Could you check a few things on this model? Use its own coordinates, in mm. Face numbers are marked on the shaded views. A direction names the side the tool comes from. Round coordinates to 2 decimals unless told otherwise and drop trailing zeros. Write each loop counter-clockwise with the first axis right and the second up, starting at its lowest first coordinate (ties: lowest second). Pieces come first, ordered by that corner, then holes. Notation, with made-up numbers: (-24.5, 17.5) -> (20.5, 17.5) arc R12 cw to (20.5, 31.5) -> close; hole circle Ø4 at (75, 78). An arc over 180 degrees is marked (long way). Answer in a Markdown table with one row per item.
from build123d import *

# Parameters (mm, degrees)
SKETCH2_R           = 25
BOSS_EXTRUDE1_DEPTH = 10
SKETCH3_R           = 17.5
BOSS_EXTRUDE3_DEPTH = 20
SKETCH4_R           = 13.5
CUT_EXTRUDE1_DEPTH  = 25
SKETCH5_W           = 13.75
SKETCH5_H           = 13.75
BOSS_EXTRUDE4_DEPTH = 100
FILLET2_R           = 2.5
FILLET3_R           = 2.5
WRAP1_START         = 12.5
WRAP1_OUTLINE_R     = 18
WRAP1_OUTLINE_R_2   = 17.5
WRAP1_DEPTH         = 6.23469337
SKETCH8_W           = 13.75
SKETCH8_H           = 13.75
CUT_EXTRUDE2_DEPTH  = 5
SKETCH8_2_W         = 13.75
SKETCH8_2_H         = 13.75
CUT_EXTRUDE3_DEPTH  = 10
SCALE1_SCALE        = 0.8


# Read off the part's stored shape, not the designer's step: Wrap1
with BuildPart() as part:
    # Sketch2 → Boss-Extrude1 (new body)
    with BuildSketch(Plane(origin=(0, 0, 0), x_dir=(1, 0, 0), z_dir=(0, 1, 0))):
        with Locations(Location((0, 0, 0), (0, 0, 270))):
            Circle(SKETCH2_R)
    extrude(amount=BOSS_EXTRUDE1_DEPTH)

    # Sketch3 → Boss-Extrude3 (add)
    with BuildSketch(Plane(origin=(0, 10, 0), x_dir=(1, 0, 0), z_dir=(0, 1, 0))):
        with Locations(Location((0, 0, 0), (0, 0, 270))):
            Circle(SKETCH3_R)
    extrude(amount=BOSS_EXTRUDE3_DEPTH)

    # Sketch4 → Cut-Extrude1 (cut)
    with BuildSketch(Plane(origin=(0, 30, 0), x_dir=(1, 0, 0), z_dir=(0, 1, 0))):
        with Locations(Location((0, 0, 0), (0, 0, 270))):
            Circle(SKETCH4_R)
    extrude(amount=-CUT_EXTRUDE1_DEPTH, mode=Mode.SUBTRACT)

    # Sketch5 → Boss-Extrude4 (add)
    with BuildSketch(Plane.XZ):
        Rectangle(SKETCH5_W, SKETCH5_H)
    extrude(amount=BOSS_EXTRUDE4_DEPTH)

    # Fillet2
    fillet2_edges = [part.edges().sort_by_distance(p)[0] for p in [
        (0, 0, -25),
        (0, 10, -25),
        (0, 10, -17.5),
    ]]
    fillet(fillet2_edges, radius=FILLET2_R)

    # Fillet3
    fillet3_edges = [part.edges().sort_by_distance(p)[0] for p in [
        (0, 30, -17.5),
    ]]
    fillet(fillet3_edges, radius=FILLET3_R)

    # Wrap1 outline → Wrap1 (add)
    with BuildSketch(Plane(origin=(0, 0, 0), x_dir=(1, 0, 0), z_dir=(0, 1, 0)).offset(WRAP1_START)):
        Circle(WRAP1_OUTLINE_R)
        Circle(WRAP1_OUTLINE_R_2, mode=Mode.SUBTRACT)
    extrude(amount=WRAP1_DEPTH)

    # Sketch8 → Cut-Extrude2 (cut)
    with BuildSketch(Plane.XZ.offset(100)):
        Rectangle(SKETCH8_W, SKETCH8_H)
    extrude(amount=-CUT_EXTRUDE2_DEPTH, mode=Mode.SUBTRACT)

    # Sketch8<2> → Cut-Extrude3 (cut)
    with BuildSketch(Plane.XZ.offset(100)):
        Rectangle(SKETCH8_2_W, SKETCH8_2_H)
    extrude(amount=-CUT_EXTRUDE3_DEPTH, mode=Mode.SUBTRACT)


with BuildPart() as part_1:
    # Scale1: scaled about (0, -12.821549585, 0)
    add(part.part.scale(SCALE1_SCALE).moved(Location((0, -2.564309917, 0))))


solid = part_1.part
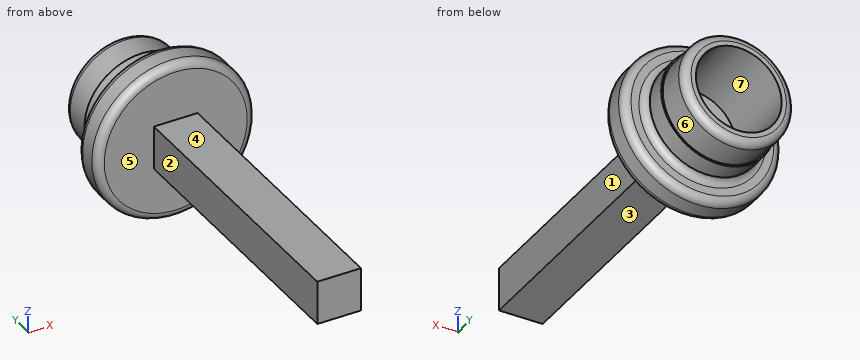
1) Imagine slicing it at C-C, the plane y = -62. Please give me the cut outline in (x, z), plus the area to 3 significant figures.
Findings:
| item | result |
|---|---|
| outline | (-5.5, -5.5) -> (5.5, -5.5) -> (5.5, 5.5) -> (-5.5, 5.5) -> close |
| area | 121 mm^2 |
2) For pin 1 (17.5 mm diameter, centred on x = 0.5, z = -2.5, fed in from +Y); pin 2 (12 mm diameter, centred on y = -45.5, z = -1, fed in from -X); pin 3 (5 mm diameter, centred on x = -9.5, z = -14, fed in from -Y); pin 4 (3 mm diameter, centred on x = -15.5, z = 9.5, fed in from +Y), each with a flat end and sliding along its axis, tell me the tip position at first contact or that it passes through.
Findings:
| item | result |
|---|---|
| pin 1 | stops at y = 21.44 |
| pin 2 | stops at x = -5.5 |
| pin 3 | stops at y = -2.56 |
| pin 4 | stops at y = 5.44 |
3) For the marked faces 1, 2 and 3, which set-ups out of +Z, -Z, +X, -X, +Y, -Y let a thin tool reach every point of the face, with its end or its side?
Findings:
| item | result |
|---|---|
| face 1 | +Z, -Z, +X, -Y |
| face 2 | +Z, -Z, -X, -Y |
| face 3 | -Z, +X, -X, -Y |
4) Thinking about a two-plate mould opening in Z: for the marked faces 4, 5, 6 and 7, which applies, +Z half, -Z half, draft (parallel to the pull), parting line (faces both ways), or undercut?
Findings:
| item | result |
|---|---|
| face 4 | +Z half |
| face 5 | draft |
| face 6 | parting line |
| face 7 | undercut |
5) Please list where these lines run through material, in increasing order: line 1 (X direction, y = 11, z = 0); line 2 (X direction, y = 13, z = 0); line 3 (Z direction, x = 9, y = 12.5).
Findings:
| item | result |
|---|---|
| line 1 | x = -14.4 to -10.8, 10.8 to 14.4 |
| line 2 | x = -14 to -10.8, 10.8 to 14 |
| line 3 | z = -10.72 to -5.97, 5.97 to 10.72 |
